Could you check a few things on this model? Use its own coordinates, in mm. A direction names the side the tool comes from. Round coordinates to 2 decimals unless told otherwise and drop trailing zeros. Loops run counter-clockwise (first coordinate to the right, second up) from the corner with the lowest first, then second, coordinate; pieces in that order, holes last. Notation, with made-up numbers: (22, 38) - (70, 38) arc R5 ccw to (70, 42) - close; hole circle Ø3 at (43, 34). An arc over 180 degrees is marked (long way). Use one line per item in the form item = value.
```python
from build123d import *

# Parameters (mm, degrees)
F0_W     = 381
F0_H     = 99.06
F1_DEPTH = 19.05
F2_R     = 43.537927
F3_W     = 330.2
F3_H     = 44.45
F4_DEPTH = 19.051
F5_R     = 21.59


with BuildPart() as f1:
    # F0 (on Front) → F1 (new body)
    with BuildSketch(Plane.XZ):
        with Locations((190.5, -49.53)):
            Rectangle(F0_W, F0_H)
    extrude(amount=F1_DEPTH)

    # F2
    f2_edges = [f1.edges().sort_by_distance(p)[0] for p in [
        (0, -9.525, -99.06),
        (381, -9.525, -99.06),
    ]]
    fillet(f2_edges, radius=F2_R)

    # F3 (on face) → F4 (cut, through all)
    with BuildSketch(Plane.XZ.offset(19.05)):
        with Locations((190.5, -49.53)):
            Rectangle(F3_W, F3_H)
    extrude(amount=-F4_DEPTH, mode=Mode.SUBTRACT)

    # F5
    f5_edges = [f1.edges().sort_by_distance(p)[0] for p in [
        (25.4, -9.525, -71.755),
        (25.4, -9.525, -27.305),
        (355.6, -9.525, -27.305),
        (355.6, -9.525, -71.755),
    ]]
    fillet(f5_edges, radius=F5_R)


solid = f1.part
```
1. For P1, Ø6, axis at y = -15, z = -68.5, coming from the -X side, with a flat end and sliding along its axis, tell me the tip position at first contact or that it passes through.
Solution:
P1 = 1.16
2. If we section it at C-C, the plane z = -31: Write out the boundary of the cut face in (x, y), plus the area to 3 significant figures.
Solution:
outline = (0, -19.05) - (34.91, -19.05) - (34.91, 0) - (0, 0) - close; (346.09, -19.05) - (381, -19.05) - (381, 0) - (346.09, 0) - close
area = 1,330 mm^2
3. If we section it at A-A, the plane x = 87: Write out the boundary of the cut face in (y, z) (3 decimals).
Solution:
outline = (-19.05, -99.06) - (0, -99.06) - (0, -71.755) - (-19.05, -71.755) - close; (-19.05, -27.305) - (0, -27.305) - (0, 0) - (-19.05, 0) - close
4. Please list where these lines run through material, in increasing order: line 1 along Z through (x, y) = (134, -13.5) (3 decimals); line 2 along X through (y, z) = (-15.25, -43); line 3 along X through (y, z) = (-6.5, -38.5).
Solution:
line_1 = -99.06 to -71.755, -27.305 to 0
line_2 = 0 to 26.22, 354.78 to 381
line_3 = 0 to 28.07, 352.93 to 381
5. If we section it at B-B, the plane y = -8: Write out the boundary of the cut face in (x, z) (3 decimals).
Solution:
outline = (0, -55.522) arc R43.538 ccw to (43.538, -99.06) - (337.462, -99.06) arc R43.538 ccw to (381, -55.522) - (381, 0) - (0, 0) - close; hole (25.4, -50.165) arc R21.59 ccw to (46.99, -71.755) - (334.01, -71.755) arc R21.59 ccw to (355.6, -50.165) - (355.6, -48.895) arc R21.59 ccw to (334.01, -27.305) - (46.99, -27.305) arc R21.59 ccw to (25.4, -48.895) - close
6. On a 3-axis mill with a long thin cutter (end or side, diameter ignored), from which of +Z, -Z, +X, -X, +Y, -Y can I reach the whole of each face in a straight line? I mean faces 4 (the face through (381, -9, -28)), 5 (the face through (349.443, -9.392, -33.797)). Say none if no direction works.
Solution:
face_4 = +Z, -Z, +X, +Y, -Y
face_5 = +Y, -Y
7. We'd pull the mould along X, two halves only. Please class faces 1 (the face through (12.42, -9.66, -85.97)), 2 (the face through (188, -9, 0)), 3 (the face through (349.108, -9.392, -65.598)): +X half, -X half, draft (parallel to the pull), parting line (faces both ways), or undercut.
Solution:
face_1 = -X half
face_2 = draft
face_3 = undercut
